Could you check a few things on this model? Use its own coordinates, in mm. A direction names the side the tool comes from. Give positions to 0.01 mm unless a question says otherwise; leave off trailing zeros. Write each loop counter-clockwise with the first axis right and the second up, starting at its lowest first coordinate (ties: lowest second). Pieces come first, ordered by that corner, then holes. Notation, with made-up numbers: (52, 25) - (66, 25) arc R25 ccw to (66, 55) - close; hole circle Ø1 at (69.5, 38.25). An arc over 180 degrees is marked (long way). Use one line per item in the form item = value.
```python
from build123d import *

# Parameters (mm, degrees)
F0_R     = 9.5
F1_DEPTH = 5
F2_R     = 5
F3_DEPTH = 9
F4_R     = 2


with BuildPart() as f1:
    # F0 (on Top) → F1 (new body)
    with BuildSketch(Plane.XY):
        Circle(F0_R)
    extrude(amount=F1_DEPTH)

    # F2 (on Top) → F3 (join)
    with BuildSketch(Plane.XY):
        Circle(F2_R)
    extrude(amount=F3_DEPTH)

    # F4
    f4_edges = [f1.edges().sort_by_distance(p)[0] for p in [
        (-9.5, 0, 0),
    ]]
    fillet(f4_edges, radius=F4_R)


solid = f1.part
```
1. Imagine slicing it at D-D, the plane z = 8.25. List the corners of the cut face in (x, y) for me, and give its area (3 significant figures).
Response values:
outline = circle Ø10 at (0, 0)
area = 78.5 mm²
2. Which directions (+Z, -Z, +X, -X, +Y, -Y) give clear straight access to the entire face, cutting with the end or side of a thin tool? Please do faces 1 (the face through (0, 0, 0)), 2 (the face through (4, -4, 5)).
Response values:
face_1 = -Z, +X, -X, +Y, -Y
face_2 = +Z
3. If I drill on line 1 (Y direction, x = -0.25, z = 2); line 2 (Z direction, x = 0.25, y = -7.5); line 3 (X direction, y = 1.25, z = 5.25), over which ranges is the centre line in solid material (lowest first)? Write a range as from..to.
Response values:
line_1 = -9.5..9.5
line_2 = 0..5
line_3 = -4.84..4.84
4. Imagine slicing it at A-A, the plane x = 0. List the corners of the cut face in (y, z) for me.
Response values:
outline = (-9.5, 2) arc R2 ccw to (-7.5, 0) - (7.5, 0) arc R2 ccw to (9.5, 2) - (9.5, 5) - (5, 5) - (5, 9) - (-5, 9) - (-5, 5) - (-9.5, 5) - close
5. Imagine slicing it at C-C, the plane z = 2.5. List the corners of the cut face in (x, y) for me.
Response values:
outline = circle Ø19 at (0, 0)
6. For pin 1 (1 mm diameter, centred on x = 4, z = 4, fed in from +Y), with a flat end and sliding along its axis, tell me the tip position at first contact or that it passes through.
Response values:
pin_1 = 8.83
